Design review of the part built by this model. Coordinates are the model's own, in mm. A direction names the side the tool comes from. Round coordinates to 2 decimals unless told otherwise and drop trailing zeros. Loops run counter-clockwise (first coordinate to the right, second up) from the corner with the lowest first, then second, coordinate; pieces in that order, holes last. Notation, with made-up numbers: (41, 87.5) - (57, 87.5) arc R9 cw to (57, 97.5) - close; hole circle Ø7 at (54, 8.5). An arc over 180 degrees is marked (long way). Use one line per item in the form item = value. Start each with the question number.
(1) Wall thickness on probe 1 along Y at (x, z) = (0, 5.5); probe 2 along X at (y, z) = (41.91, 7.75); probe 3 along Y at (x, z) = (-0.5, 8): over which ranges is each line inside the solid? List them lowest first. Write a range as [from, to].
(2) For pin 1 (4 mm diameter, centred on x = -1, y = 35, fed in from +Z) (3 decimals); pin 2 (6 mm diameter, centred on x = 0, y = 41.91, fed in from +Z); pin 3 (3 mm diameter, centred on x = -2, y = 7.5, fed in from +Z) (3 decimals), all flat-tipped, find the tip position at first contact; note any pin that passes through.
(3) The part is to be moulded in two halves that separate along Y. For faces 3 (the flat face through (-3, 26, 9.525)), 4 (the cylindrical face through (5.44, 49.85, 4.83)), 5 (the cylindrical face through (2.896, 7.856, 1.61)), say which applies: released by +Y, released by -Y, zero draft, split by the parting line, or undercut.
(4) Machinability: for faces 1 (the flat face through (-1, 3, 3.175)), 2 (the cylindrical face through (1.25, 18.255, 4.829)), which of the approach directions +Z, -Z, +X, -X, +Y, -Y give a long, thin tool a straight path to every point of the face, cutting with its end or side? Answer none if there is none.
(5) We need section B-B, the plane y = 33.02. Write out the cut boundary in (x, z) (3 decimals).
(6) We need section C-C, the plane z = 5. Give the number of separate pieces and of enclosed holes in the cut face, then the cut area to 3 significant figures.
(7) We need section A-A, the plane x = 0. Write out the cut boundary in (y, z) (1 decimal).
Autodesk Inventor part; units mm, degrees
ref_plane "YZ Plane" through (0, 0, 0) normal (1, 0, 0) x (0, 1, 0)
ref_plane "XZ Plane" through (0, 0, 0) normal (0, 1, 0) x (-1, 0, 0)
ref_plane "XY Plane" through (0, 0, 0) normal (0, 0, 1) x (1, 0, 0)
sketch "Sketch1" plane through (0, 0, 0) normal (0, 0, 1) x (1, 0, 0)
  line L0 (-6.35, 0) -> (6.35, 0)
  line L1 (6.35, 0) -> (6.35, 50.8)
  line L2 (6.35, 50.8) -> (-6.35, 50.8)
  line L3 (-6.35, 50.8) -> (-6.35, 0)
  point P0 (0, 0)
  dimension "d6" = 50.8
  dimension "d7" = 12.7
  dimension "d22" = 6.35
extrude "Stock Bar" add sketch "Sketch1" along normal blind 9.525
sketch "Sketch4" plane through (0, 0, 0) normal (0, 0, -1) x (-1, 0, 0)
  line L0 (6.35, 0) -> (-6.35, 0)
  line L1 (-6.35, 0) -> (-6.35, 50.8)
  point P0 (0, 0)
  point P1 (0, 6.35)
  dimension "d13" = 6.35
  dimension "d14" = 6.35
hole "Motor Hole" at (0, 6.35, 0) direction (0, 0, 1) diameter 6.5278 end through all
sketch "Sketch6" plane through (0, 0, 9.525) normal (0, 0, 1) x (1, 0, 0)
  circle A0 centre (0, 6.35) radius 3.2639
  circle A1 centre (0, 6.35) radius 4.7625
  point P0 (0, 0)
  dimension "d25" = 9.525
extrude "Motor Hole Secondary" cut sketch "Sketch6" against normal blind 6.35
sketch "Sketch5" plane through (0, 0, 9.525) normal (0, 0, 1) x (1, 0, 0)
  line L0 (-6.35, 50.8) -> (-6.35, 0)
  line L1 (-6.35, 25.4) -> (6.35, 25.4) construction
  line L2 (6.35, 0) -> (6.35, 50.8)
  point P0 (0, 0)
fillet "Round Edges" radius 3.175 4 edges at (-6.35, 50.8, 4.7625) (6.35, 50.8, 4.7625) (6.35, 0, 4.7625) (-6.35, 0, 4.7625)
pattern_linear "Mounting Holes" count 5 spacing 8.89 along (0, 1, 0) of "Motor Hole"
sketch "Sketch7" plane through (0, 0, 9.525) normal (0, 0, 1) x (1, 0, 0)
  line L0 (-6.35, 47.625) -> (-6.35, 3.175)
  line L1 (-6.35, 25.4) -> (6.35, 25.4) construction
  line L2 (6.35, 3.175) -> (6.35, 47.625)
  line L3 (0, 25.4) -> (0, 0) construction
  line L4 (-3.175, 0) -> (3.175, 0)
properties part number "Arm" material "Aluminum 6061"
Data:
q1.probe_1 = [0, 1.59], [11.11, 11.98], [18.5, 20.87], [27.39, 29.76], [36.28, 38.65], [45.17, 50.8]
q1.probe_2 = [-6.35, -3.26], [3.26, 6.35]
q1.probe_3 = [0, 1.61], [11.09, 12.01], [18.47, 20.9], [27.36, 29.79], [36.25, 38.68], [45.14, 50.8]
q2.pin_1 = 9.525
q2.pin_2 = through
q2.pin_3 = 3.175
q3.face_3 = zero draft
q3.face_4 = released by +Y
q3.face_5 = undercut
q4.face_1 = +Z
q4.face_2 = +Z, -Z
q5.outline = (-6.35, 0) - (-3.264, 0) - (-3.264, 9.525) - (-6.35, 9.525) - close; (3.264, 0) - (6.35, 0) - (6.35, 9.525) - (3.264, 9.525) - close
q6.separate_pieces = 1
q6.enclosed_holes = 5
q6.area = 431 mm^2
q7.outline = (0, 0) - (3.1, 0) - (3.1, 3.2) - (1.6, 3.2) - (1.6, 9.5) - (0, 9.5) - close; (9.6, 0) - (12, 0) - (12, 9.5) - (11.1, 9.5) - (11.1, 3.2) - (9.6, 3.2) - close; (18.5, 0) - (20.9, 0) - (20.9, 9.5) - (18.5, 9.5) - close; (27.4, 0) - (29.8, 0) - (29.8, 9.5) - (27.4, 9.5) - close; (36.3, 0) - (38.6, 0) - (38.6, 9.5) - (36.3, 9.5) - close; (45.2, 0) - (50.8, 0) - (50.8, 9.5) - (45.2, 9.5) - close
